Autodesk Inventor part; units mm, degrees
ref_plane "YZ Plane" through (0, 0, 0) normal (1, 0, 0) x (0, 1, 0)
ref_plane "XZ Plane" through (0, 0, 0) normal (0, 1, 0) x (-1, 0, 0)
ref_plane "XY Plane" through (0, 0, 0) normal (0, 0, 1) x (1, 0, 0)
sketch "Sketch1" plane through (0, 0, 0) normal (0, 0, 1) x (1, 0, 0)
  circle A0 centre (0, 0) radius 20
  dimension "d0" = 40
extrude "Extrusion1" add sketch "Sketch1" along normal blind 5
sketch "Sketch2" plane through (0, 0, 0) normal (0, 0, -1) x (-1, 0, 0)
  circle A0 centre (0, 0) radius 15
  dimension "d3" = 30
extrude "Extrusion2" add sketch "Sketch2" along normal blind 44.45
sketch "Sketch3" plane through (0, 0, 5) normal (0, 0, 1) x (1, 0, 0)
  circle A0 centre (0, 0) radius 4.5
  dimension "d6" = 9
extrude "Extrusion3" cut sketch "Sketch3" against normal through all
sketch "Sketch4" plane through (0, 0, 5) normal (0, 0, 1) x (1, 0, 0)
  circle A0 centre (0, 0) radius 4.5
  line L0 (-4, 2.0616) -> (-4, 19.5959)
  circle A1 centre (0, 0) radius 20
  line L1 (4, 2.0616) -> (4, 19.5959)
  line L2 (0, -28) -> (0, 28)
  arc A2 (4, 2.0616) -> (-4, 2.0616) centre (0, 0) ccw
  arc A3 (0, -20) -> (-4, 19.5959) centre (0, 0) ccw
  dimension "d11" = 4
extrude "Extrusion4" cut sketch "Sketch4" against normal through all contours A0 L2 A1 L1 | A0 L0 A1 L2 picked at (1.3394, 14.7583) picked at (-1.3394, 14.7583)
properties part number "wallPlug"
For this review, take the finished solid that the model builds, in its own axes (mm). A direction names the side the tool comes from. Round coordinates to 2 decimals unless told otherwise and drop trailing zeros. Write each loop counter-clockwise with the first axis right and the second up, starting at its lowest first coordinate (ties: lowest second). Pieces come first, ordered by that corner, then holes. Notation, with made-up numbers: (63.5, 50) - (86.5, 50) arc R19 ccw to (86.5, 67) - close; hole circle Ø3 at (43.5, 84). An arc over 180 degrees is marked (long way). Write each question's results on one line, items separated by ' | '.
Item 1: For faces 4 (the face through (-0.1, -4.5, -19.4)), 5 (the face through (-0.603, -14.988, -21.914)), 6 (the face through (4, 9, -19)), list the 3-axis set-ups (+Z, -Z, +X, -X, +Y, -Y) from which the entire face can be reached by the end or side of a thin tool; tool diameter is ignored.
Calculated:
face 4: +Z, -Z | face 5: -Z | face 6: +Z, -Z, +Y
Item 2: For pin 1 (1 mm diameter, centred on y = -5.5, z = -21.5, fed in from -X); pin 2 (2 mm diameter, centred on y = 6.5, z = -28, fed in from -X); pin 3 (14 mm diameter, centred on y = 10.5, z = -13.5, fed in from +X); pin 4 (7 mm diameter, centred on x = 0, y = 0, fed in from +Z), all flat-tipped, find the tip position at first contact; note any pin that passes through.
Calculated:
pin 1: stops at x = -14.14 | pin 2: stops at x = -13.96 | pin 3: stops at x = 14.59 | pin 4: passes through
Item 3: Draft analysis for pull direction X (two halves, no side actions). For faces 1 (the face through (-4, 9, -19)), 2 (the face through (-3, -15, 0)), 3 (the face through (0.823, -19.983, 2.465)), state which applies: pulls with the +X half, pulls with the -X half, needs draft (parallel to the pull), parting line crosses it, or undercut.
Calculated:
face 1: undercut | face 2: needs draft | face 3: parting line crosses it
Item 4: To check wall thickness, follow line 1 along X through (y, z) = (0, -14); line 2 along Z through (x, y) = (5, 15); line 3 along Y through (x, z) = (0, -28). State the ranges of each line that lie inside material, in increasing order. Write a range as from..to.
Calculated:
line 1: x = -15..-4.5, 4.5..15 | line 2: z = 0..5 | line 3: y = -15..-4.5
Item 5: Take a section at C-C on y = 16. State the section outline as (x, z) points.
Calculated:
outline: (-12, 0) - (-4, 0) - (-4, 5) - (-12, 5) - close; (4, 0) - (12, 0) - (12, 5) - (4, 5) - close
Item 6: Take a section at D-D on x = 9.5. State the section outline as (y, z) points, then the cut area to 3 significant figures.
Calculated:
outline: (-17.6, 0) - (-11.61, 0) - (-11.61, -44.45) - (11.61, -44.45) - (11.61, 0) - (17.6, 0) - (17.6, 5) - (-17.6, 5) - close | area: 1,210 mm^2
Item 7: Take a section at A-A on y = 0. State the section outline as (x, z) points.
Calculated:
outline: (-20, 0) - (-15, 0) - (-15, -44.45) - (-4.5, -44.45) - (-4.5, 5) - (-20, 5) - close; (4.5, -44.45) - (15, -44.45) - (15, 0) - (20, 0) - (20, 5) - (4.5, 5) - close
Item 8: Take a section at B-B on x = 0. State the section outline as (y, z) points.
Calculated:
outline: (-20, 0) - (-15, 0) - (-15, -44.45) - (-4.5, -44.45) - (-4.5, 5) - (-20, 5) - close
